Print and shaded views of the part. All mm, measured from the part's lowest x, y and z. Coordinates: 2 decimals unless noted, no trailing zeros. Write each loop counter-clockwise with the first axis right and the second up, starting at its lowest first coordinate (ties: lowest second). Pieces come first, ordered by that corner, then holes. Notation, with made-up numbers: (2.25, 86.5) -> (53.25, 86.5) arc R36 cw to (53.25, 120.5) -> close; hole circle Ø7 at (-23, 70). An arc over 180 degrees is marked (long way). Write item = value, one per line.
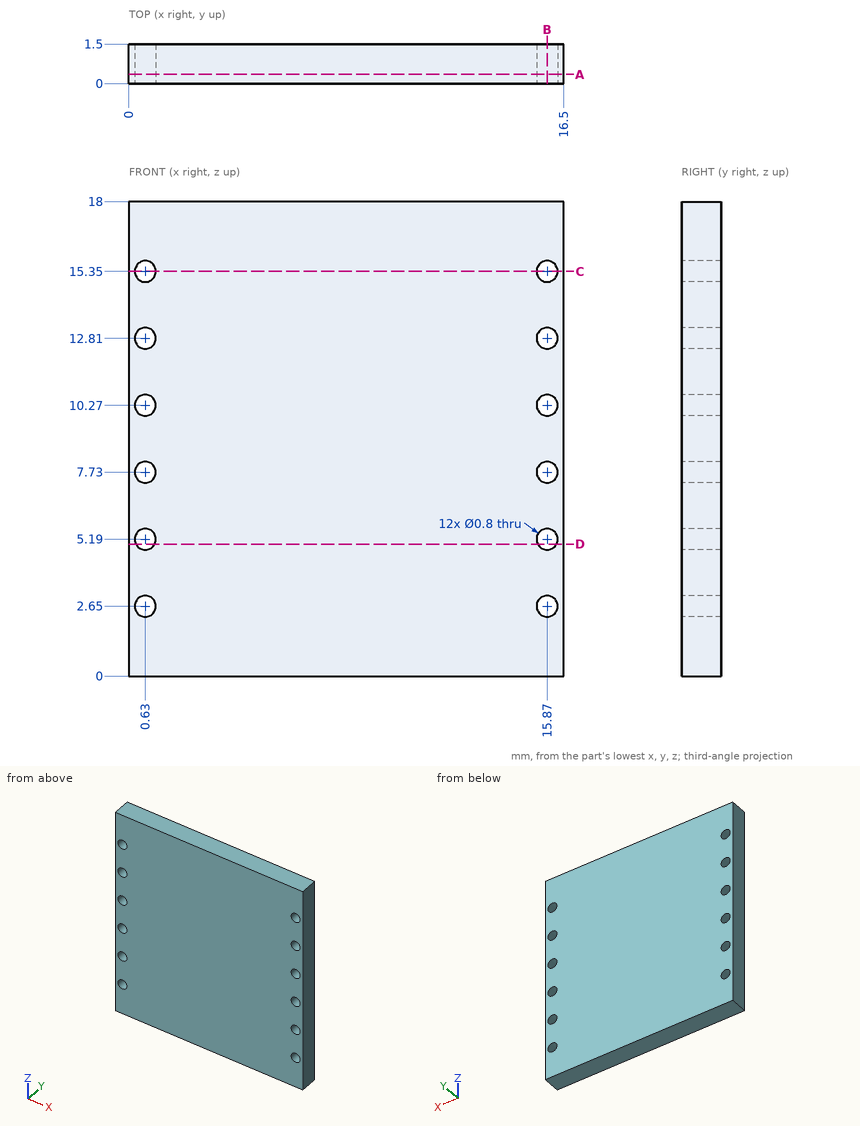
Q1. Saw through at B-B on x = 15.87. Give the cut face in (y, z), and give its area (3 significant figures).
Model answer:
outline = (0, 0) -> (1.5, 0) -> (1.5, 2.25) -> (0, 2.25) -> close; (0, 3.05) -> (1.5, 3.05) -> (1.5, 4.79) -> (0, 4.79) -> close; (0, 5.59) -> (1.5, 5.59) -> (1.5, 7.33) -> (0, 7.33) -> close; (0, 8.13) -> (1.5, 8.13) -> (1.5, 9.87) -> (0, 9.87) -> close; (0, 10.67) -> (1.5, 10.67) -> (1.5, 12.41) -> (0, 12.41) -> close; (0, 13.21) -> (1.5, 13.21) -> (1.5, 14.95) -> (0, 14.95) -> close; (0, 15.75) -> (1.5, 15.75) -> (1.5, 18) -> (0, 18) -> close
area = 19.8 mm²
Q2. Probe line 1 (X direction, y = 1.1, z = 10.27); line 2 (X direction, y = 1.35, z = 3). List the from-to ranges inside material, lowest first. Write a range as from..to.
Model answer:
line_1 = 0..0.23, 1.03..15.47, 16.27..16.5
line_2 = 0..0.44, 0.82..15.68, 16.06..16.5
Q3. Saw through at C-C on z = 15.35. Give the cut face in (x, y), and give its area (4 significant figures).
Model answer:
outline = (0, 0) -> (0.23, 0) -> (0.23, 1.5) -> (0, 1.5) -> close; (1.03, 0) -> (15.47, 0) -> (15.47, 1.5) -> (1.03, 1.5) -> close; (16.27, 0) -> (16.5, 0) -> (16.5, 1.5) -> (16.27, 1.5) -> close
area = 22.35 mm²
Q4. Saw through at D-D on z = 5. Give the cut face in (x, y), and give its area (3 significant figures).
Model answer:
outline = (0, 0) -> (0.28, 0) -> (0.28, 1.5) -> (0, 1.5) -> close; (0.98, 0) -> (15.52, 0) -> (15.52, 1.5) -> (0.98, 1.5) -> close; (16.22, 0) -> (16.5, 0) -> (16.5, 1.5) -> (16.22, 1.5) -> close
area = 22.6 mm²
Q5. Saw through at A-A on y = 0.35. Count the separate pieces of the cut face and the enclosed holes in it, and give its area (3 significant figures).
Model answer:
separate_pieces = 1
enclosed_holes = 12
area = 291 mm²
